Job drawing, mm, ordinate dimensions from the low corner. One solid piece. A direction names the side the tool comes from. Coordinates: 2 decimals unless noted, no trailing zeros. Loops run counter-clockwise (first coordinate to the right, second up) from the corner with the lowest first, then second, coordinate; pieces in that order, holes last. Notation, with made-up numbers: (-29, -11.5) - (14, -11.5) arc R24 ccw to (14, 25.5) - close; hole circle Ø9 at (68, 86.25). An arc over 180 degrees is marked (long way). Use a Markdown table: item, result. Add a question column.
1. Drop flat-ended pins along their axis: pin 1 (6 mm diameter, centred on x = 10.5, y = 5, fed in from -Z); pin 2 (9 mm diameter, centred on x = 60, z = 36, fed in from -Y). Give the stop position or say it passes through.
2. Band-saw the part on C-C, the plane z = 8. Give the cut face in (x, y).
3. Wall check: probe 1 along Z at (x, y) = (24, 16); probe 2 along X at (y, z) = (17.25, 57.5); probe 3 along Y at (x, z) = (67.5, 45). Give the ranges that are in metal, low to high. Write a range as [from, to].
4. Band-saw the part on B-B, the plane y = 2.75. Give the cut face in (x, z).
5. 3-axis set-ups, long thin cutter, end or side, ignore diameter. For the marked faces 1 and 2: which of +Z, -Z, +X, -X, +Y, -Y reach the whole face in a straight line?
6. Band-saw the part on A-A, the plane x = 60. Give the cut face in (y, z).
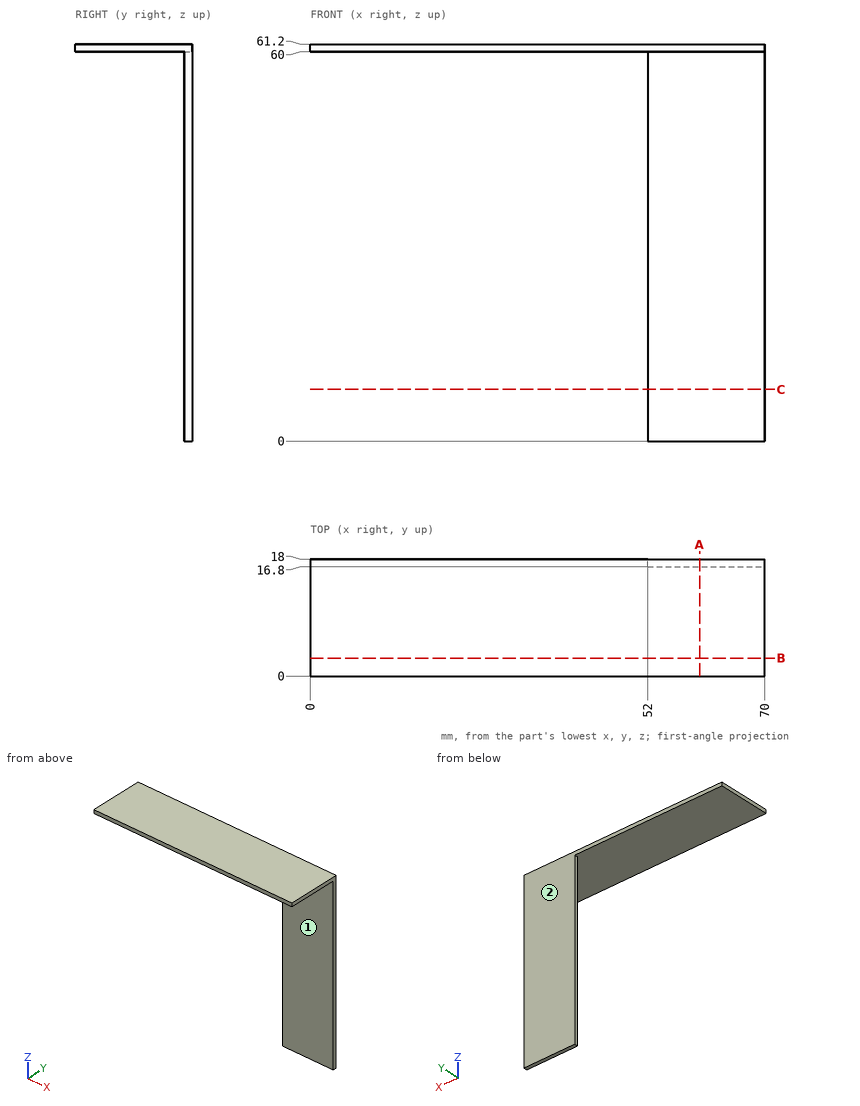
Geometry check:
| question | item | result |
|---|---|---|
| 1 | pin 1 | stops at z = 60 |
| 1 | pin 2 | stops at y = 16.8 |
| 2 | outline | (52, 16.8) - (70, 16.8) - (70, 18) - (52, 18) - close |
| 3 | probe 1 | z = [60, 61.2] |
| 3 | probe 2 | x = [52, 70] |
| 3 | probe 3 | y = [16.8, 18] |
| 4 | outline | (0, 60) - (70, 60) - (70, 61.2) - (0, 61.2) - close |
| 5 | face 1 | -Z, +X, -X, -Y |
| 5 | face 2 | +Z, -Z, +X, -X, +Y |
| 6 | outline | (0, 60) - (16.8, 60) - (16.8, 0) - (18, 0) - (18, 61.2) - (0, 61.2) - close |
